Source: CAD feature listing. Evaluate the final solid. Frame: model axes, mm. A direction names the side the tool comes from. Round coordinates to 2 decimals unless told otherwise and drop trailing zeros. Write each loop counter-clockwise with the first axis right and the second up, starting at its lowest first coordinate (ties: lowest second). Pieces come first, ordered by that corner, then holes. Notation, with made-up numbers: M -30,26 L 27,26 A31 ccw 27,50 Z; hole C 58.25,54 d7. An arc over 180 degrees is marked long. Answer in a Markdown table with one row per item. Add a question column.
Item 1: Contact query for flat-ended pins moving along their axis: pin 1 (0.5 mm diameter, centred on x = 5, y = 9, fed in from -Z); pin 2 (0.7 mm diameter, centred on x = 7.5, y = 12, fed in from +Z); pin 3 (2 mm diameter, centred on x = 7, z = 1.5, fed in from +Y). Output: stop coordinate, or through.
Item 2: Cut plane A-A on y = 11. Return loops of the section in (x, z), and give its area (3 significant figures).
Item 3: Set-up query: faces 5 (the face through (8.89, 1, 0)), 6 (the face through (0.32, -3, 2)), 7 (the face through (0, 1, -1.25)), 8 (the face through (5, 1, 1.25)), 9 (the face through (-0.32, -3, 2)). Return all of +Z, -Z, +X, -X, +Y, -Y with unobstructed straight access to the full face (end or side cutting, diameter ignored); none if empty.
Item 4: Material intervals for probe 1 along X at (y, z) = (13.25, 0); probe 2 along Y at (x, z) = (4.75, -0.5); probe 3 along Z at (x, y) = (-0.25, 9), sorted ascending.
Item 5: Cut plane C-C on x = 1. Return loops of the section in (y, z), and give its area (3 significant figures).
Item 6: Cut plane B-B on z = 3.75. Return loops of the section in (x, y), and give its area (3 significant figures).
Item 7: Mould query, pull axis X, two halves, no side actions, for faces 1 (the face through (7.94, -3, 2)), 2 (the face through (8, 1, 1.25)), 3 (the face through (-1.27, 1, 0)), 4 (the face through (4.76, -3, 2)). Classes: released by +X, released by -X, zero draft, split by the parting line, or undercut.
from build123d import *
from OCP.BRepFilletAPI import BRepFilletAPI_MakeChamfer

# Parameters (mm, degrees)
BOSS_EXTRUDE1_DEPTH         = 2.29
SKETCH3_W                   = 0.64
SKETCH3_H                   = 0.64
CHAMFER3_SIZE               = 0.5
CHAMFER3_SIZE2              = 0.133974596
LPATTERN1_COUNT             = 4
LPATTERN1_PITCH             = 2.54
CHAMFER3_OF_LPATTERN1_SIZE  = 0.5
CHAMFER3_OF_LPATTERN1_SIZE2 = 0.133974596


with BuildPart() as part:
    # Sketch1 → Boss-Extrude1 (new body)
    with BuildSketch(Plane(origin=(0, 0, 0), x_dir=(1, 0, 0), z_dir=(0, 1, 0))):
        Polygon((-0.77, 1.25), (0.77, 1.25), (1.25, 0.75), (1.27, 0.75), (1.27, -0.75), (1.25, -0.75), (0.77, -1.25), (-0.77, -1.25), (-1.25, -0.75), (-1.27, -0.75), (-1.27, 0.75), (-1.25, 0.75), align=None)
    boss_extrude1 = extrude(amount=BOSS_EXTRUDE1_DEPTH)

    # Sweep1: sweep along a path in Sketch2
    with BuildLine(Plane(origin=(0, 0, 0), x_dir=(0, 0, -1), z_dir=(1, 0, 0))) as sweep1_path:
        Line((0, 17.12), (0, -0.408142235))
        ThreePointArc((0, -0.408142235), (-0.152240935, -1.1735091), (-0.585786438, -1.822355798))
        Line((-0.585786438, -1.822355798), (-5.26343064, -6.5))
    # Sketch3 → Sweep1 (sweep)
    with BuildSketch(Plane(origin=(0, 17.12, 0), x_dir=(1, 0, 0), z_dir=(0, 1, 0))):
        Rectangle(SKETCH3_W, SKETCH3_H)
    sweep1 = sweep(path=sweep1_path.line)

    # Chamfer3: one chamfer whose edges measure the first distance from different faces: ONE call of the kernel's chamfer builder (chamfer() names one face for all edges)
    chamfer3_edges_1 = [part.edges().sort_by_distance(p)[0] for p in [
        (0.32, 17.12, 0),
    ]]
    chamfer3_side_1 = [part.faces().sort_by_distance(p)[0] for p in [
        (0.32, 9.705, 0),
    ]]
    chamfer3_edges_2 = [part.edges().sort_by_distance(p)[0] for p in [
        (0, 17.12, -0.32),
    ]]
    chamfer3_side_2 = [part.faces().sort_by_distance(p)[0] for p in [
        (0, 9.705, -0.32),
    ]]
    chamfer3_edges_3 = [part.edges().sort_by_distance(p)[0] for p in [
        (-0.32, 17.12, 0),
    ]]
    chamfer3_side_3 = [part.faces().sort_by_distance(p)[0] for p in [
        (-0.32, 9.705, 0),
    ]]
    chamfer3_edges_4 = [part.edges().sort_by_distance(p)[0] for p in [
        (0, 17.12, 0.32),
    ]]
    chamfer3_side_4 = [part.faces().sort_by_distance(p)[0] for p in [
        (0, 9.705, 0.32),
    ]]
    chamfer3 = BRepFilletAPI_MakeChamfer(part.part.solid().wrapped)
    for e in chamfer3_edges_1:
        chamfer3.Add(CHAMFER3_SIZE, CHAMFER3_SIZE2, e.wrapped, chamfer3_side_1[0].wrapped)  # the first distance lies on this face
    for e in chamfer3_edges_2:
        chamfer3.Add(CHAMFER3_SIZE, CHAMFER3_SIZE2, e.wrapped, chamfer3_side_2[0].wrapped)  # the first distance lies on this face
    for e in chamfer3_edges_3:
        chamfer3.Add(CHAMFER3_SIZE, CHAMFER3_SIZE2, e.wrapped, chamfer3_side_3[0].wrapped)  # the first distance lies on this face
    for e in chamfer3_edges_4:
        chamfer3.Add(CHAMFER3_SIZE, CHAMFER3_SIZE2, e.wrapped, chamfer3_side_4[0].wrapped)  # the first distance lies on this face
    add(Compound.cast(chamfer3.Shape()), mode=Mode.REPLACE)

    # LPattern1: Boss-Extrude1, Sweep1 ×4
    with Locations(*[(i * LPATTERN1_PITCH, 0, 0) for i in range(1, LPATTERN1_COUNT)]):
        add(boss_extrude1)
        add(sweep1)

    # Chamfer3 of LPattern1: one chamfer whose edges measure the first distance from different faces: ONE call of the kernel's chamfer builder (chamfer() names one face for all edges)
    chamfer3_of_lpattern1_edges_1 = [part.edges().sort_by_distance(p)[0] for p in [
        (2.86, 17.12, 0),
    ]]
    chamfer3_of_lpattern1_side_1 = [part.faces().sort_by_distance(p)[0] for p in [
        (2.86, 9.705, 0),
    ]]
    chamfer3_of_lpattern1_edges_2 = [part.edges().sort_by_distance(p)[0] for p in [
        (2.54, 17.12, -0.32),
    ]]
    chamfer3_of_lpattern1_side_2 = [part.faces().sort_by_distance(p)[0] for p in [
        (2.54, 9.705, -0.32),
    ]]
    chamfer3_of_lpattern1_edges_3 = [part.edges().sort_by_distance(p)[0] for p in [
        (2.22, 17.12, 0),
    ]]
    chamfer3_of_lpattern1_side_3 = [part.faces().sort_by_distance(p)[0] for p in [
        (2.22, 9.705, 0),
    ]]
    chamfer3_of_lpattern1_edges_4 = [part.edges().sort_by_distance(p)[0] for p in [
        (2.54, 17.12, 0.32),
    ]]
    chamfer3_of_lpattern1_side_4 = [part.faces().sort_by_distance(p)[0] for p in [
        (2.54, 9.705, 0.32),
    ]]
    chamfer3_of_lpattern1_edges_5 = [part.edges().sort_by_distance(p)[0] for p in [
        (5.4, 17.12, 0),
    ]]
    chamfer3_of_lpattern1_side_5 = [part.faces().sort_by_distance(p)[0] for p in [
        (5.4, 9.705, 0),
    ]]
    chamfer3_of_lpattern1_edges_6 = [part.edges().sort_by_distance(p)[0] for p in [
        (5.08, 17.12, -0.32),
    ]]
    chamfer3_of_lpattern1_side_6 = [part.faces().sort_by_distance(p)[0] for p in [
        (5.08, 9.705, -0.32),
    ]]
    chamfer3_of_lpattern1_edges_7 = [part.edges().sort_by_distance(p)[0] for p in [
        (4.76, 17.12, 0),
    ]]
    chamfer3_of_lpattern1_side_7 = [part.faces().sort_by_distance(p)[0] for p in [
        (4.76, 9.705, 0),
    ]]
    chamfer3_of_lpattern1_edges_8 = [part.edges().sort_by_distance(p)[0] for p in [
        (5.08, 17.12, 0.32),
    ]]
    chamfer3_of_lpattern1_side_8 = [part.faces().sort_by_distance(p)[0] for p in [
        (5.08, 9.705, 0.32),
    ]]
    chamfer3_of_lpattern1_edges_9 = [part.edges().sort_by_distance(p)[0] for p in [
        (7.94, 17.12, 0),
    ]]
    chamfer3_of_lpattern1_side_9 = [part.faces().sort_by_distance(p)[0] for p in [
        (7.94, 9.705, 0),
    ]]
    chamfer3_of_lpattern1_edges_10 = [part.edges().sort_by_distance(p)[0] for p in [
        (7.62, 17.12, -0.32),
    ]]
    chamfer3_of_lpattern1_side_10 = [part.faces().sort_by_distance(p)[0] for p in [
        (7.62, 9.705, -0.32),
    ]]
    chamfer3_of_lpattern1_edges_11 = [part.edges().sort_by_distance(p)[0] for p in [
        (7.3, 17.12, 0),
    ]]
    chamfer3_of_lpattern1_side_11 = [part.faces().sort_by_distance(p)[0] for p in [
        (7.3, 9.705, 0),
    ]]
    chamfer3_of_lpattern1_edges_12 = [part.edges().sort_by_distance(p)[0] for p in [
        (7.62, 17.12, 0.32),
    ]]
    chamfer3_of_lpattern1_side_12 = [part.faces().sort_by_distance(p)[0] for p in [
        (7.62, 9.705, 0.32),
    ]]
    chamfer3_of_lpattern1 = BRepFilletAPI_MakeChamfer(part.part.solid().wrapped)
    for e in chamfer3_of_lpattern1_edges_1:
        chamfer3_of_lpattern1.Add(CHAMFER3_OF_LPATTERN1_SIZE, CHAMFER3_OF_LPATTERN1_SIZE2, e.wrapped, chamfer3_of_lpattern1_side_1[0].wrapped)  # the first distance lies on this face
    for e in chamfer3_of_lpattern1_edges_2:
        chamfer3_of_lpattern1.Add(CHAMFER3_OF_LPATTERN1_SIZE, CHAMFER3_OF_LPATTERN1_SIZE2, e.wrapped, chamfer3_of_lpattern1_side_2[0].wrapped)  # the first distance lies on this face
    for e in chamfer3_of_lpattern1_edges_3:
        chamfer3_of_lpattern1.Add(CHAMFER3_OF_LPATTERN1_SIZE, CHAMFER3_OF_LPATTERN1_SIZE2, e.wrapped, chamfer3_of_lpattern1_side_3[0].wrapped)  # the first distance lies on this face
    for e in chamfer3_of_lpattern1_edges_4:
        chamfer3_of_lpattern1.Add(CHAMFER3_OF_LPATTERN1_SIZE, CHAMFER3_OF_LPATTERN1_SIZE2, e.wrapped, chamfer3_of_lpattern1_side_4[0].wrapped)  # the first distance lies on this face
    for e in chamfer3_of_lpattern1_edges_5:
        chamfer3_of_lpattern1.Add(CHAMFER3_OF_LPATTERN1_SIZE, CHAMFER3_OF_LPATTERN1_SIZE2, e.wrapped, chamfer3_of_lpattern1_side_5[0].wrapped)  # the first distance lies on this face
    for e in chamfer3_of_lpattern1_edges_6:
        chamfer3_of_lpattern1.Add(CHAMFER3_OF_LPATTERN1_SIZE, CHAMFER3_OF_LPATTERN1_SIZE2, e.wrapped, chamfer3_of_lpattern1_side_6[0].wrapped)  # the first distance lies on this face
    for e in chamfer3_of_lpattern1_edges_7:
        chamfer3_of_lpattern1.Add(CHAMFER3_OF_LPATTERN1_SIZE, CHAMFER3_OF_LPATTERN1_SIZE2, e.wrapped, chamfer3_of_lpattern1_side_7[0].wrapped)  # the first distance lies on this face
    for e in chamfer3_of_lpattern1_edges_8:
        chamfer3_of_lpattern1.Add(CHAMFER3_OF_LPATTERN1_SIZE, CHAMFER3_OF_LPATTERN1_SIZE2, e.wrapped, chamfer3_of_lpattern1_side_8[0].wrapped)  # the first distance lies on this face
    for e in chamfer3_of_lpattern1_edges_9:
        chamfer3_of_lpattern1.Add(CHAMFER3_OF_LPATTERN1_SIZE, CHAMFER3_OF_LPATTERN1_SIZE2, e.wrapped, chamfer3_of_lpattern1_side_9[0].wrapped)  # the first distance lies on this face
    for e in chamfer3_of_lpattern1_edges_10:
        chamfer3_of_lpattern1.Add(CHAMFER3_OF_LPATTERN1_SIZE, CHAMFER3_OF_LPATTERN1_SIZE2, e.wrapped, chamfer3_of_lpattern1_side_10[0].wrapped)  # the first distance lies on this face
    for e in chamfer3_of_lpattern1_edges_11:
        chamfer3_of_lpattern1.Add(CHAMFER3_OF_LPATTERN1_SIZE, CHAMFER3_OF_LPATTERN1_SIZE2, e.wrapped, chamfer3_of_lpattern1_side_11[0].wrapped)  # the first distance lies on this face
    for e in chamfer3_of_lpattern1_edges_12:
        chamfer3_of_lpattern1.Add(CHAMFER3_OF_LPATTERN1_SIZE, CHAMFER3_OF_LPATTERN1_SIZE2, e.wrapped, chamfer3_of_lpattern1_side_12[0].wrapped)  # the first distance lies on this face
    add(Compound.cast(chamfer3_of_lpattern1.Shape()), mode=Mode.REPLACE)


solid = part.part
Results below:
| question | item | result |
|---|---|---|
| 1 | pin 1 | z = -0.32 |
| 1 | pin 2 | z = 0.32 |
| 1 | pin 3 | y = 2.29 |
| 2 | outline | M -0.32,-0.32 L 0.32,-0.32 L 0.32,0.32 L -0.32,0.32 Z; M 2.22,-0.32 L 2.86,-0.32 L 2.86,0.32 L 2.22,0.32 Z; M 4.76,-0.32 L 5.4,-0.32 L 5.4,0.32 L 4.76,0.32 Z; M 7.3,-0.32 L 7.94,-0.32 L 7.94,0.32 L 7.3,0.32 Z |
| 2 | area | 1.64 mm2 |
| 3 | face 5 | +Z, -Z, +X, +Y, -Y |
| 3 | face 6 | +Z, -Z, -Y |
| 3 | face 7 | -Z, +X, -X, +Y, -Y |
| 3 | face 8 | +Z, +X, -X, +Y |
| 3 | face 9 | +Z, -Z, -X, -Y |
| 4 | probe 1 | -0.32 to 0.32, 2.22 to 2.86, 4.76 to 5.4, 7.3 to 7.94 |
| 4 | probe 2 | 0 to 2.29 |
| 4 | probe 3 | -0.32 to 0.32 |
| 5 | outline | M 0,-1.01 L 2.29,-1.01 L 2.29,1.01 L 0,1.01 Z |
| 5 | area | 4.63 mm2 |
| 6 | outline | M -0.32,-5.44 L 0.32,-5.44 L 0.32,-4.53 L -0.32,-4.53 Z; M 2.22,-5.44 L 2.86,-5.44 L 2.86,-4.53 L 2.22,-4.53 Z; M 4.76,-5.44 L 5.4,-5.44 L 5.4,-4.53 L 4.76,-4.53 Z; M 7.3,-5.44 L 7.94,-5.44 L 7.94,-4.53 L 7.3,-4.53 Z |
| 6 | area | 2.32 mm2 |
| 7 | face 1 | released by +X |
| 7 | face 2 | zero draft |
| 7 | face 3 | released by -X |
| 7 | face 4 | undercut |
